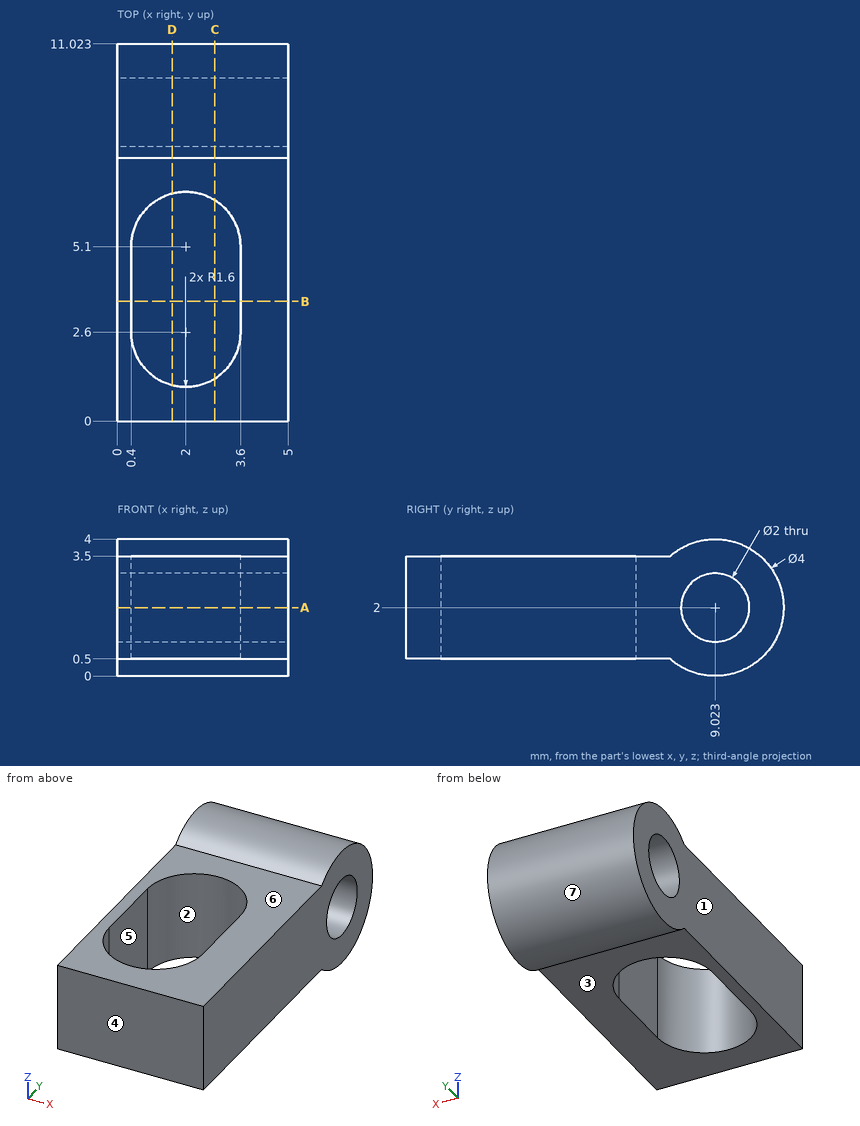
Can you work these out from the drawing? Everything is in mm from the part's minimum corner. A direction names the side the tool comes from. Coordinates: 2 decimals unless noted, no trailing zeros. Write each loop counter-clockwise with the first axis right and the second up, starting at its lowest first coordinate (ties: lowest second). Pieces come first, ordered by that corner, then holes. Notation, with made-up numbers: (39.25, 26.25) - (71.25, 26.25) arc R30 ccw to (71.25, 62.25) - close; hole circle Ø7 at (35, -31). An arc over 180 degrees is marked (long way). Use a Markdown table: item, result.
Q1. Imagine slicing it at A-A (z = 2). List the corners of the cut face in (x, y) for me.
Geometry check:
| item | result |
|---|---|
| outline | (0, 0) - (5, 0) - (5, 8.02) - (0, 8.02) - close; (0, 10.02) - (5, 10.02) - (5, 11.02) - (0, 11.02) - close; hole (0.4, 2.6) arc R1.6 ccw to (3.6, 2.6) - (3.6, 5.1) arc R1.6 ccw to (0.4, 5.1) - close |
Q2. Imagine slicing it at D-D (x = 1.6). List the corners of the cut face in (y, z) for me.
Geometry check:
| item | result |
|---|---|
| outline | (0, 0.5) - (1.05, 0.5) - (1.05, 3.5) - (0, 3.5) - close; (6.65, 0.5) - (7.7, 0.5) arc R2 ccw (long way) to (7.7, 3.5) - (6.65, 3.5) - close; hole circle Ø2 at (9.02, 2) |
Q3. Imagine slicing it at C-C (x = 2.85). List the corners of the cut face in (y, z) for me.
Geometry check:
| item | result |
|---|---|
| outline | (0, 0.5) - (1.24, 0.5) - (1.24, 3.5) - (0, 3.5) - close; (6.46, 0.5) - (7.7, 0.5) arc R2 ccw (long way) to (7.7, 3.5) - (6.46, 3.5) - close; hole circle Ø2 at (9.02, 2) |
Q4. Which directions (+Z, -Z, +X, -X, +Y, -Y) give clear straight access to the entire face, cutting with the end or side of a thin tool? Please do the marked faces 1, 2 and 3.
Geometry check:
| item | result |
|---|---|
| face 1 | +Z, -Z, -X, +Y, -Y |
| face 2 | +Z, -Z |
| face 3 | -Z, +X, -X, -Y |
Q5. Imagine slicing it at B-B (y = 3.5). List the corners of the cut face in (x, z) for me.
Geometry check:
| item | result |
|---|---|
| outline | (0, 0.5) - (0.4, 0.5) - (0.4, 3.5) - (0, 3.5) - close; (3.6, 0.5) - (5, 0.5) - (5, 3.5) - (3.6, 3.5) - close |
Q6. Please list where these lines run through material, in increasing order: L1, parallel to Y at x = 0.85, z = 1.1; L2, parallel to X at y = 3.25, z = 3.2; L3, parallel to Y at x = 1.8, z = 2.
Geometry check:
| item | result |
|---|---|
| L1 | y = 0 to 1.49, 6.21 to 8.59, 9.46 to 10.81 |
| L2 | x = 0 to 0.4, 3.6 to 5 |
| L3 | y = 0 to 1.01, 6.69 to 8.02, 10.02 to 11.02 |
Q7. I'm going to push flat-ended pins straight in: pin 1 Ø2 at (x, y) = (0.5, 3.5) entering from -Z; pin 2 Ø2 at (y, z) = (4, 2) entering from -X; pin 3 Ø1.8 at (y, z) = (9.02, 2) entering from +X. Where does each tip first touch, or does it pass through?
Geometry check:
| item | result |
|---|---|
| pin 1 | stops at z = 0.5 |
| pin 2 | stops at x = 0 |
| pin 3 | passes through |
Q8. Thinking about a two-plate mould opening in Y: for the marked faces 4, 5, 6 and 7, which applies, +Y half, -Y half, draft (parallel to the pull), parting line (faces both ways), or undercut?
Geometry check:
| item | result |
|---|---|
| face 4 | -Y half |
| face 5 | undercut |
| face 6 | draft |
| face 7 | parting line |
